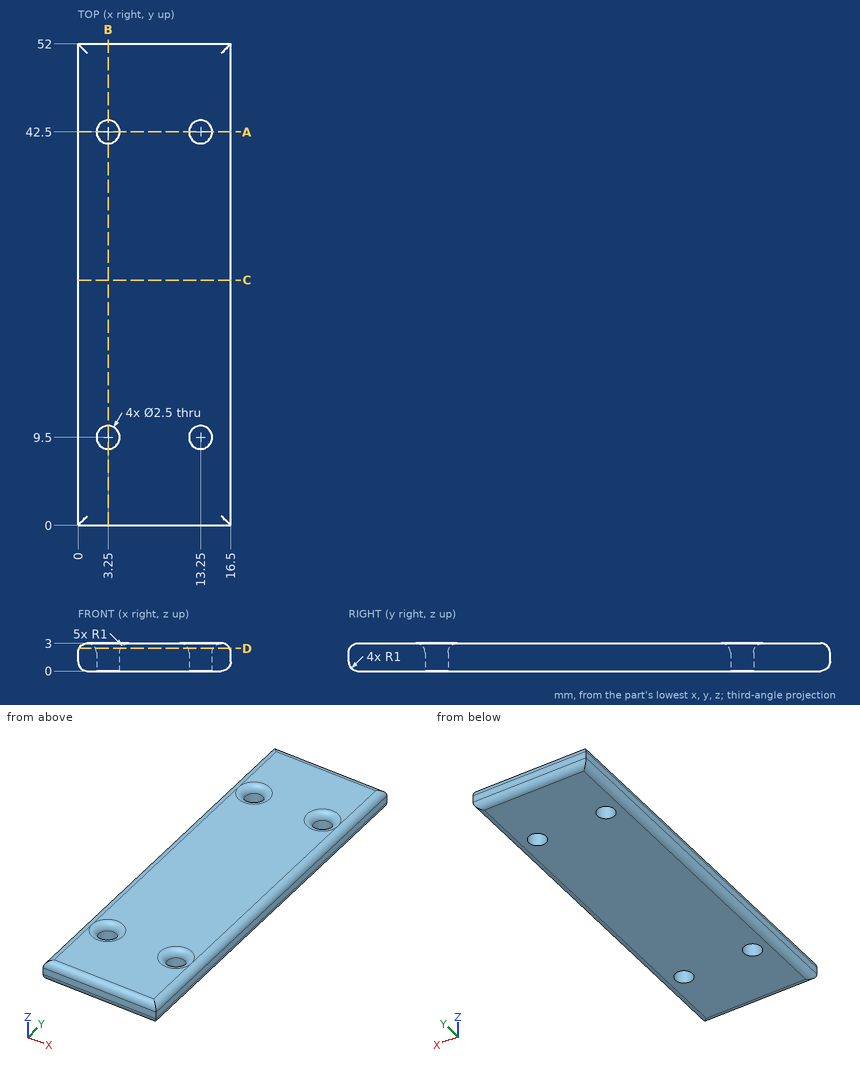
Can you work these out from the drawing? Everything is in mm from the part's minimum corner. Round coordinates to 2 decimals unless told otherwise and drop trailing zeros. Write each loop counter-clockwise with the first axis right and the second up, starting at its lowest first coordinate (ties: lowest second). Pieces come first, ordered by that corner, then holes. Notation, with made-up numbers: M 79,58 L 122,58 A33 ccw 122,95 Z; hole C 75.5,85 d4. An arc over 180 degrees is marked long. Use a Markdown table: item, result.
Item 1: If I drill on line 1 along Y through (x, z) = (3.25, 1.55); line 2 along Y through (x, z) = (14, 1.1); line 3 along X through (y, z) = (50, 2.2), over which ranges is the centre line in solid material (lowest first)? Write a range as [from, to].
Found:
| item | result |
|---|---|
| line 1 | y = [0, 8.25], [10.75, 41.25], [43.75, 52] |
| line 2 | y = [0, 8.5], [10.5, 41.5], [43.5, 52] |
| line 3 | x = [0.02, 16.48] |
Item 2: I want a section at B-B (x = 3.25). List the corners of the cut face in (y, z) for me, and give its area (3 significant figures).
Found:
| item | result |
|---|---|
| outline | M 0,1 A1 ccw 1,0 L 8.25,0 L 8.25,2 A1 ccw 7.25,3 L 1,3 A1 ccw 0,2 Z; M 10.75,0 L 41.25,0 L 41.25,2 A1 ccw 40.25,3 L 11.75,3 A1 ccw 10.75,2 Z; M 43.75,0 L 51,0 A1 ccw 52,1 L 52,2 A1 ccw 51,3 L 44.75,3 A1 ccw 43.75,2 Z |
| area | 139 mm2 |
Item 3: I want a section at D-D (z = 2.45). List the corners of the cut face in (x, y) for me, and give its area (3 significant figures).
Found:
| item | result |
|---|---|
| outline | M 0.11,0.11 L 16.39,0.11 L 16.39,51.89 L 0.11,51.89 Z; hole C 3.25,9.5 d2.71; hole C 3.25,42.5 d2.71; hole C 13.25,9.5 d2.71; hole C 13.25,42.5 d2.71 |
| area | 820 mm2 |
Item 4: I want a section at A-A (y = 42.5). State how many separate pieces and enclosed holes the cut face has, and give its area (3 significant figures).
Found:
| item | result |
|---|---|
| separate pieces | 3 |
| enclosed holes | 0 |
| area | 32.8 mm2 |
Item 5: For pin 1 Ø3 at (x, y) = (13.25, 9.5) entering from +Z, with a flat end and sliding along its axis, tell me the tip position at first contact or that it passes through.
Found:
| item | result |
|---|---|
| pin 1 | stops at z = 2.66 |
Item 6: I want a section at C-C (y = 26.5). List the corners of the cut face in (x, z) for me, and give its area (3 significant figures).
Found:
| item | result |
|---|---|
| outline | M 0,1 A1 ccw 1,0 L 15.5,0 A1 ccw 16.5,1 L 16.5,2 A1 ccw 15.5,3 L 1,3 A1 ccw 0,2 Z |
| area | 48.6 mm2 |
